from build123d import *

# Parameters (mm, degrees)
BOX015_W               = 120
BOX015_H               = 30
BOX015_DEPTH           = 84
CYLINDER069_R          = 2.5
CYLINDER069_DEPTH      = 10
CYLINDER070_R          = 2.5
CYLINDER070_DEPTH      = 10
CYLINDER071_R          = 2.5
CYLINDER071_DEPTH      = 10
CYLINDER072_R          = 2.5
CYLINDER072_DEPTH      = 10
CYLINDER068_R          = 2.5
CYLINDER068_DEPTH      = 10
CYLINDER073_R          = 2.5
CYLINDER073_DEPTH      = 10
BOX009_W               = 240
BOX009_H               = 5
BOX009_DEPTH           = 24
BOX010_W               = 140
BOX010_H               = 5
BOX010_DEPTH           = 38
BOX011_W               = 140
BOX011_H               = 5
BOX011_DEPTH           = 42
CUT008_PLACEMENT_ANGLE = 270


with BuildPart() as gatewaycut001:
    # Box015 → Box015 (new body)
    with BuildSketch(Plane(origin=(-75, -3.2, -75), x_dir=(1, 0, 0), z_dir=(0, 0, 1))):
        with Locations((60, 15)):
            Rectangle(BOX015_W, BOX015_H)
    extrude(amount=BOX015_DEPTH)


with BuildPart() as cylinder069:
    # Cylinder069 → Cylinder069 (new body)
    with BuildSketch(Plane(origin=(115, 0, -31), x_dir=(1, 0, 0), z_dir=(0, -1, 0))):
        Circle(CYLINDER069_R)
    extrude(amount=CYLINDER069_DEPTH)


with BuildPart() as cylinder070:
    # Cylinder070 → Cylinder070 (new body)
    with BuildSketch(Plane(origin=(-80, 0, -31), x_dir=(1, 0, 0), z_dir=(0, -1, 0))):
        Circle(CYLINDER070_R)
    extrude(amount=CYLINDER070_DEPTH)


with BuildPart() as cylinder071:
    # Cylinder071 → Cylinder071 (new body)
    with BuildSketch(Plane(origin=(50, 0, -31), x_dir=(1, 0, 0), z_dir=(0, -1, 0))):
        Circle(CYLINDER071_R)
    extrude(amount=CYLINDER071_DEPTH)


with BuildPart() as cylinder072:
    # Cylinder072 → Cylinder072 (new body)
    with BuildSketch(Plane(origin=(-45.75, 0, -56.3), x_dir=(1, 0, 0), z_dir=(0, -1, 0))):
        Circle(CYLINDER072_R)
    extrude(amount=CYLINDER072_DEPTH)


with BuildPart() as cylinder068:
    # Cylinder068 → Cylinder068 (new body)
    with BuildSketch(Plane(origin=(-115, 0, -31), x_dir=(1, 0, 0), z_dir=(0, -1, 0))):
        Circle(CYLINDER068_R)
    extrude(amount=CYLINDER068_DEPTH)


with BuildPart() as m3heatsetinserts003:
    # Cylinder073 → Cylinder073 (new body)
    with BuildSketch(Plane(origin=(-45.75, 0, -1.3), x_dir=(1, 0, 0), z_dir=(0, -1, 0))):
        Circle(CYLINDER073_R)
    extrude(amount=CYLINDER073_DEPTH)

    # Fusion025: union Cylinder069, Cylinder070, Cylinder071, Cylinder072, Cylinder068
    add(cylinder069.part)
    add(cylinder070.part)
    add(cylinder071.part)
    add(cylinder072.part)
    add(cylinder068.part)


with BuildPart() as m3heatsetinserts003_1:
    # Fusion025 placement: moved
    add(m3heatsetinserts003.part.moved(Location((0, 5.1, 0))))


with BuildPart() as cube007:
    # Box009 → Box009 (new body)
    with BuildSketch(Plane(origin=(-120, 0, -43), x_dir=(1, 0, 0), z_dir=(0, 0, 1))):
        with Locations((120, 2.5)):
            Rectangle(BOX009_W, BOX009_H)
    extrude(amount=BOX009_DEPTH)


with BuildPart() as cube008:
    # Box010 → Box010 (new body)
    with BuildSketch(Plane(origin=(-85, 0, -19), x_dir=(1, 0, 0), z_dir=(0, 0, 1))):
        with Locations((70, 2.5)):
            Rectangle(BOX010_W, BOX010_H)
    extrude(amount=BOX010_DEPTH)


with BuildPart() as mainbase001:
    # Box011 → Box011 (new body)
    with BuildSketch(Plane(origin=(-85, 0, -85), x_dir=(1, 0, 0), z_dir=(0, 0, 1))):
        with Locations((70, 2.5)):
            Rectangle(BOX011_W, BOX011_H)
    extrude(amount=BOX011_DEPTH)

    # Fusion020: union Cube007, Cube008
    add(cube007.part)
    add(cube008.part)

    # Cut007: cut M3HeatSetInserts003
    add(m3heatsetinserts003_1.part, mode=Mode.SUBTRACT)

    # Cut008: cut GatewayCut001
    add(gatewaycut001.part, mode=Mode.SUBTRACT)


with BuildPart() as mainbase001_1:
    # Cut008 placement: moved
    add(mainbase001.part.rotate(Axis((0, 0, 0), (1, 0, 0)), CUT008_PLACEMENT_ANGLE))


solid = mainbase001_1.part
Part model, mm, in its own coordinate system. A direction names the side the tool comes from. Round coordinates to 2 decimals unless told otherwise and drop trailing zeros. Write each loop counter-clockwise with the first axis right and the second up, starting at its lowest first coordinate (ties: lowest second). Pieces come first, ordered by that corner, then holes. Notation, with made-up numbers: (-35.5, -20.75) - (-26.5, -20.75) arc R23 ccw to (-26.5, 13.25) - close; hole circle Ø2 at (9, 18). An arc over 180 degrees is marked (long way). Use CSV: the item, a comma, the result in double quotes.
Item 1: Flat gauge pins, fed straight in: P1, Ø2, axis at y = -72.5, z = -2, coming from the +X side; P2, Ø6, axis at x = 41.5, y = -48, coming from the -Z side; P3, Ø1.5, axis at x = -109.5, z = -2, coming from the +Y side; P4, Ø1.5, axis at y = -8.5, z = -2, coming from the -X side. Where does each tip first touch, or does it go through?
Results list:
P1,"stops at x = 55"
P2,"passes through"
P3,"stops at y = -19"
P4,"stops at x = -85"
Item 2: Wall check: L1, parallel to X at y = -31, z = -2.2; L2, parallel to Y at x = -40.5, z = -0.7; L3, parallel to X at y = 4, z = -1.85. Give the ranges that are in metal, low to high.
Results list:
L1,"x = -120 to -117.5, -112.5 to -82.5, -77.5 to -75, 45 to 47.5, 52.5 to 112.5, 117.5 to 120"
L2,"y = -85 to -75, 9 to 19"
L3,"x = -85 to -75, 45 to 55"
Item 3: Tool access for faces 4 (the flat face through (-2, 12, 0)), 5 (the flat face through (55, -64, -2)), 6 (the flat face through (-16, -75, -3)), 7 (the flat face through (-103, -19, -3)), 8 (the flat face through (55, 0, -2)): list every direction of +Z, -Z, +X, -X, +Y, -Y with a clear straight run to the whole face (end or side of a thin tool).
Results list:
face 4,"+Z, +X, -X, +Y, -Y"
face 5,"+Z, -Z, +X, -Y"
face 6,"+Z, -Z"
face 7,"+Z, -Z, -X, +Y"
face 8,"+Z, -Z, +X, +Y"
Item 4: Pull direction X, two halves, no side cores. Call faces 1 (the flat face through (-103, -43, -3)), 2 (the cylindrical face through (-112.615, -30.249, -2.535)), 3 (the flat face through (-85, -64, -2)): pulls with the +X half, pulls with the -X half, needs draft (parallel to the pull), parting line crosses it, or undercut.
Results list:
face 1,"needs draft"
face 2,"undercut"
face 3,"pulls with the -X half"
Item 5: Slice it at C-C, the plane y = -31. Write the cut outline in (x, z), then the cut area to 3 significant figures.
Results list:
outline,"(-120, -5) - (-117.5, -5) - (-117.5, 0) - (-120, 0) - close; (-112.5, -5) - (-82.5, -5) - (-82.5, 0) - (-112.5, 0) - close; (-77.5, -5) - (-75, -5) - (-75, 0) - (-77.5, 0) - close; (45, -5) - (47.5, -5) - (47.5, 0) - (45, 0) - close; (52.5, -5) - (112.5, -5) - (112.5, 0) - (52.5, 0) - close; (117.5, -5) - (120, -5) - (120, 0) - (117.5, 0) - close"
area,"500 mm²"
Item 6: Slice it at B-B, the plane z = -3.9. Write the cut outline in (x, y).
Results list:
outline,"(-120, -43) - (-85, -43) - (-85, -85) - (55, -85) - (55, -43) - (120, -43) - (120, -19) - (55, -19) - (55, 19) - (-85, 19) - (-85, -19) - (-120, -19) - close; hole circle Ø5 at (-115, -31); hole circle Ø5 at (-80, -31); hole (-75, -75) - (45, -75) - (45, 9) - (-75, 9) - close; hole circle Ø5 at (50, -31); hole circle Ø5 at (115, -31)"
Item 7: Slice it at A-A, the plane x = -44. Write the cut outline in (y, z), then the cut area to 3 significant figures.
Results list:
outline,"(-85, -5) - (-75, -5) - (-75, 0) - (-85, 0) - close; (9, -5) - (19, -5) - (19, 0) - (9, 0) - close"
area,"100 mm²"
Item 8: Slice it at D-D, the plane x = -80. Write the cut outline in (y, z).
Results list:
outline,"(-85, -5) - (-33.5, -5) - (-33.5, 0) - (-85, 0) - close; (-28.5, -5) - (19, -5) - (19, 0) - (-28.5, 0) - close"
